CAD build for the part. Positions are in the model's coordinates, mm. A direction names the side the tool comes from. Round coordinates to 2 decimals unless told otherwise and drop trailing zeros. Loops run counter-clockwise (first coordinate to the right, second up) from the corner with the lowest first, then second, coordinate; pieces in that order, holes last. Notation, with made-up numbers: M -37.5,-37 L -1.5,-37 A10 cw -1.5,-24 Z; hole C -9,-32.5 d7. An arc over 180 degrees is marked long. Use one line per item in the form item = value.
from build123d import *

# Parameters (mm, degrees)
SKETCH1_W                    = 7.7
SKETCH1_H                    = 10
BASE_FLANGE1_DEPTH           = 1
EDGE_FLANGE1_STRIP_W         = 5.4732
EDGE_FLANGE1_STRIP_H         = 1
EDGE_FLANGE1_STRIP_CUT_DEPTH = 10
EDGE_FLANGE1_DEPTH           = 10
SKETCH11_W                   = 23
SKETCH11_H                   = 10
TAB1_DEPTH                   = 1
FILLET1_R                    = 1
FILLET2_R                    = 2
SKETCH15_R                   = 1.75
CUT_EXTRUDE1_DEPTH           = 22.626141588
EDGE_FLANGE2_STRIP_W         = 5.4732
EDGE_FLANGE2_STRIP_H         = 1
EDGE_FLANGE2_STRIP_CUT_DEPTH = 10
EDGE_FLANGE2_DEPTH           = 10
CUT_EXTRUDE2_DEPTH           = 33.86335345
FILLET3_R                    = 2


# Sheet-metal steps are written as plain solids
with BuildPart() as part:
    # Sketch1 → Base-Flange1 (new body)
    with BuildSketch(Plane(origin=(0, 0, 0), x_dir=(1, 0, 0), z_dir=(0, 1, 0))):
        with Locations((3.85, 0)):
            Rectangle(SKETCH1_W, SKETCH1_H)
    extrude(amount=-BASE_FLANGE1_DEPTH)

    # Edge-Flange1 strip (across the edge) → Edge-Flange1 strip cut (cut)
    with BuildSketch(Plane(origin=(7.7, 0, 5), x_dir=(-1, 0, 0), z_dir=(0, 0, -1))):
        with Locations((-2, -0.5)):
            Rectangle(EDGE_FLANGE1_STRIP_W, EDGE_FLANGE1_STRIP_H)
    extrude(amount=EDGE_FLANGE1_STRIP_CUT_DEPTH, mode=Mode.SUBTRACT)

    # Edge-Flange1 section (across the edge) → Edge-Flange1 (add)
    with BuildSketch(Plane(origin=(7.7, 0, 5), x_dir=(-1, 0, 0), z_dir=(0, 0, -1))):
        with BuildLine():
            Line((-1, 0.7366), (-1, 4))
            Line((-1, 4), (0, 4))
            Line((0, 4), (0, 0.7366))
            ThreePointArc((0, 0.7366), (0.215745145, 0.215745145), (0.7366, 0))
            Line((0.7366, 0), (0.7366, -1))
            ThreePointArc((0.7366, -1), (-0.491361636, -0.491361636), (-1, 0.7366))
        make_face()
    extrude(amount=EDGE_FLANGE1_DEPTH)

    # Sketch11 → Tab1 (add)
    with BuildSketch(Plane(origin=(8.7, 0, 0), x_dir=(0, 0, -1), z_dir=(1, 0, 0))):
        with Locations((2.5, 9)):
            Rectangle(SKETCH11_W, SKETCH11_H)
    extrude(amount=-TAB1_DEPTH)

    # Fillet1
    fillet1_edges = [part.edges().sort_by_distance(p)[0] for p in [
        (8.2, 4, 5),
        (8.2, 4, -5),
    ]]
    fillet(fillet1_edges, radius=FILLET1_R)

    # Fillet2
    fillet2_edges = [part.edges().sort_by_distance(p)[0] for p in [
        (8.2, 14, -14),
        (8.2, 4, -14),
    ]]
    fillet(fillet2_edges, radius=FILLET2_R)

    # Sketch15 → Cut-Extrude1 (cut, through all)
    with BuildSketch(Plane(origin=(8.7, 0, 0), x_dir=(0, 0, -1), z_dir=(1, 0, 0))):
        with Locations(Location((9, 9, 0), (0, 0, 90))):
            Circle(SKETCH15_R)
    extrude(amount=-CUT_EXTRUDE1_DEPTH, mode=Mode.SUBTRACT)

    # Edge-Flange2 strip (across the edge) → Edge-Flange2 strip cut (cut)
    with BuildSketch(Plane(origin=(8.7, 14, 9), x_dir=(0, 0, -1), z_dir=(0, -1, 0))):
        with Locations((-1, -0.5)):
            Rectangle(EDGE_FLANGE2_STRIP_W, EDGE_FLANGE2_STRIP_H)
    extrude(amount=EDGE_FLANGE2_STRIP_CUT_DEPTH, mode=Mode.SUBTRACT)

    # Edge-Flange2 section (across the edge) → Edge-Flange2 (add)
    with BuildSketch(Plane(origin=(8.7, 14, 9), x_dir=(0, 0, -1), z_dir=(0, -1, 0))):
        with BuildLine():
            Line((0, 0.7366), (0, 11.3))
            Line((0, 11.3), (1, 11.3))
            Line((1, 11.3), (1, 0.7366))
            ThreePointArc((1, 0.7366), (1.215745145, 0.215745145), (1.7366, 0))
            Line((1.7366, 0), (1.7366, -1))
            ThreePointArc((1.7366, -1), (0.508638364, -0.491361636), (0, 0.7366))
        make_face()
    extrude(amount=EDGE_FLANGE2_DEPTH)

    # Sketch23 → Cut-Extrude2 (cut, through all)
    with BuildSketch(Plane(origin=(0, 0, 8), x_dir=(-1, 0, 0), z_dir=(0, 0, -1))):
        with BuildLine():
            Line((-15.75, 10.65), (-14.25, 10.65))
            ThreePointArc((-14.25, 10.65), (-12.6, 9), (-14.25, 7.35))
            Line((-14.25, 7.35), (-15.75, 7.35))
            ThreePointArc((-15.75, 7.35), (-17.4, 9), (-15.75, 10.65))
        make_face()
    extrude(amount=-CUT_EXTRUDE2_DEPTH, mode=Mode.SUBTRACT)

    # Fillet3
    fillet3_edges = [part.edges().sort_by_distance(p)[0] for p in [
        (20, 14, 8.5),
        (20, 4, 8.5),
    ]]
    fillet(fillet3_edges, radius=FILLET3_R)

    # Mirror1: part across plane


with BuildPart() as part_1:
    add(part.part)
    add(part.part.mirror(Plane(origin=(0, -1, -5), x_dir=(0, 0, 1), z_dir=(-1, 0, 0))))


solid = part_1.part
1. Tool access for faces 4 (the face through (0.7, -0.5, -5)), 5 (the face through (-8.7, 7, -3)), 6 (the face through (8.2, 9.07, 8.48)), 7 (the face through (8.7, 7, -3)), 8 (the face through (7.7, 7, -3)): list every direction of +Z, -Z, +X, -X, +Y, -Y with a clear straight run to the whole face (end or side of a thin tool).
Completed:
face_4 = -Z, +X, -X, -Y
face_5 = -Z, -X, +Y, -Y
face_6 = +Z, +Y, -Y
face_7 = -Z, +X, +Y, -Y
face_8 = +Z, -Z, +Y
2. Cut at D-D on z = -3.5. Write the cut outline in (x, y), and give its area (3 significant figures).
Completed:
outline = M -8.7,0.74 A1.74 ccw -6.96,-1 L 6.96,-1 A1.74 ccw 8.7,0.74 L 8.7,14 L 7.7,14 L 7.7,0.74 A0.74 cw 6.96,0 L -6.96,0 A0.74 cw -7.7,0.74 L -7.7,14 L -8.7,14 Z
area = 44.3 mm2
3. Probe line 1 along X through (y, z) = (6, -3); line 2 along Z through (x, y) = (13, 5); line 3 along Z through (x, y) = (-8.5, 9). List the from-to ranges inside material, lowest first. Write a range as from..to.
Completed:
line_1 = -8.7..-7.7, 7.7..8.7
line_2 = 8..9
line_3 = -14..-10.75, -7.25..8.73
4. Cut at A-A on z = -9. Write the cut outline in (x, y).
Completed:
outline = M -8.7,4 L -7.7,4 L -7.7,7.25 L -8.7,7.25 Z; M -8.7,10.75 L -7.7,10.75 L -7.7,14 L -8.7,14 Z; M 7.7,4 L 8.7,4 L 8.7,7.25 L 7.7,7.25 Z; M 7.7,10.75 L 8.7,10.75 L 8.7,14 L 7.7,14 Z
5. Cut at C-C on y = 10.25. State how many separate pieces and enclosed holes the cut face has, and give its area (3 significant figures).
Completed:
separate_pieces = 6
enclosed_holes = 0
area = 55.3 mm2
6. Cut at B-B on y = 1.75. Write the cut outline in (x, z), and give its area (3 significant figures).
Completed:
outline = M -8.7,-5 L -7.7,-5 L -7.7,5 L -8.7,5 Z; M 7.7,-5 L 8.7,-5 L 8.7,5 L 7.7,5 Z
area = 20.0 mm2
7. Pull direction Y, two halves, no side cores. Call faces 1 (the face through (8.18, -0.5, 0.07)), 2 (the face through (20, 9, 8.5)), 3 (the face through (15, 7.35, 8.5)): +Y half, -Y half, draft (parallel to the pull), parting line (faces both ways), or undercut.
Completed:
face_1 = -Y half
face_2 = draft
face_3 = undercut
8. Drop flat-ended pins along their axis: P1, Ø3, axis at x = -1.5, y = 0, coming from the -Z side; P2, Ø5, axis at x = -3, z = -3, coming from the +Y side; P3, Ø3, axis at y = 4, z = -0.5, coming from the +X side. Give the stop position or say it passes through.
Completed:
P1 = -5
P2 = 0
P3 = 8.7
